Part model, mm, in its own coordinate system. A direction names the side the tool comes from. Round coordinates to 2 decimals unless told otherwise and drop trailing zeros.
1) Drop a flat-ended pin along its axis: P1, Ø1.5, axis at y = -2.5, z = 14, coming from the -X side. Give the stop position or say it passes through.
2) Mould opens along Y. For faces 4 (the flat face through (-2.642, 1.562, 18.784)), 5 (the conical face through (-0.14, 0.13, 13.52)), 6 (the flat face through (1.5, -1.4, 0)) say: +Y half, -Y half, draft (parallel to the pull), parting line (faces both ways), or undercut.
3) 3-axis set-ups, long thin cutter, end or side, ignore diameter. For faces 1 (the cylindrical face through (0.632, -1.525, 31.661)), 2 (the cylindrical face through (1.725, -0.358, 6.439)), 3 (the flat face through (0, 3.175, 19)): which of +Z, -Z, +X, -X, +Y, -Y reach the whole face in a straight line?
4) Probe line 1 (Y direction, x = 0, z = 35.5); line 2 (X direction, y = 0.75, z = 2); line 3 (X direction, y = -1.25, z = 3). List the from-to ranges inside material, lowest first.
Autodesk Inventor part; units mm, degrees
ref_plane "Work Plane1" through (-1.711, 0.0003, 0) normal (0, 1, 0) x (1, 0, 0)
ref_plane "Work Plane2" through (0.1135, 0.0003, 19.05) normal (0, 0, -1) x (-1, 0, 0)
ref_plane "YZ Plane" through (0, 0, 0) normal (1, 0, 0) x (0, 1, 0)
sketch "Sketch1" plane through (0, 0, 0) normal (0, 0, 1) x (1, 0, 0)
  line L0 (1.9552, -3.1747) -> (-1.711, -3.1747)
  line L1 (-1.711, -3.1747) -> (-3.5441, 0.0003)
  line L2 (-3.5441, 0.0003) -> (-1.711, 3.1753)
  line L3 (-1.711, 3.1753) -> (1.9552, 3.1753)
  line L4 (1.9552, 3.1753) -> (3.7883, 0.0003)
  line L5 (3.7883, 0.0003) -> (1.9552, -3.1747)
  point P0 (0.1221, 0.0003)
  dimension "d0" = 6.35
extrude "Extrusion1" add sketch "Sketch1" along normal blind 38.1
ref_plane "Work Plane1" through (-1.711, 0.0003, 0) normal (0, 1, 0) x (1, 0, 0)
sketch "Sketch3" plane through (-1.711, 0.0003, 0) normal (0, 1, 0) x (1, 0, 0)
  line L0 (-1.3251, 0) -> (4.9741, 0)
  line L1 (5.4821, -0.508) -> (5.4821, -37.592)
  line L2 (-1.8331, -37.592) -> (-1.8331, -0.508)
  line L3 (-1.8331, -0.508) -> (-1.3251, 0)
  line L4 (4.9741, 0) -> (5.4821, -0.508)
  line L5 (-1.8331, 0) -> (-1.8331, -38.1)
  line L6 (3.6662, 0) -> (5.4993, 0)
  line L7 (1.8245, 0) -> (1.8245, -38.1)
  line L8 (0, -38.1) -> (-1.8331, -38.1)
  line L9 (5.4993, -38.1) -> (3.6662, -38.1)
  line L10 (3.6662, -38.1) -> (0, -38.1)
  line L11 (-1.3251, -38.1) -> (-1.8331, -37.592)
  line L12 (4.9741, -38.1) -> (5.4821, -37.592)
  point P0 (-1.8331, 0)
  point P1 (5.4821, 0)
  point P2 (5.4821, -38.1)
  dimension "d5" = 0.508
  dimension "d6" = 0.508
  dimension "d7" = 0.508
  dimension "d8" = 0.508
  dimension "d16" = 0
  dimension "d46" = 0.508
  dimension "d47" = 0.508
  dimension "d48" = 0.508
  dimension "d49" = 0.508
revolve "Revolution1" cut sketch "Sketch3" angle 360 about axis through (0.1135, 0.0003, 0) along (0, 0, 1) keep common part contours L0 L4 L1 L12 L9 L10 L7
sketch "Sketch6" plane through (0.1135, 0.0003, 0) normal (0, 0, -1) x (-1, 0, 0)
  circle A0 centre (0, 0) radius 3.1496
hole "Hole3" at (0.1135, 0.0003, 0) direction (0, 0, 1) diameter 3.302 depth 12.7 tip angle 118
sketch "Sketch7" plane through (0, 0, 38.1) normal (0, 0, 1) x (1, 0, 0)
  point P0 (0, 0)
hole "Hole4" at (0, 0, 38.1) direction (0, 0, -1) diameter 3.302 depth 12.7 tip angle 118
ref_plane "Work Plane2" through (0.1135, 0.0003, 19.05) normal (0, 0, -1) x (-1, 0, 0)
properties part number "1.5 inch Standoff" material "Steel"
Reported:
1. P1: stops at x = -2.53
2. face 4: +Y half
2. face 5: undercut
2. face 6: draft
3. face 1: +Z
3. face 2: -Z
3. face 3: +Z, -Z, +X, -X, +Y
4. line 1: y = -3.17 to -1.65, 1.65 to 3.18
4. line 2: x = -3.11 to -1.36, 1.58 to 3.36
4. line 3: x = -2.82 to -0.96, 1.19 to 3.07
